```python
from build123d import *

# Parameters (mm, degrees)
SKETCH2_W           = 38.1
SKETCH2_H           = 38.1
SKETCH3_R           = 10
BOSS_EXTRUDE1_DEPTH = 38.1
FILLET1_R           = 40
SKETCH4_W           = 7.62
SKETCH4_H           = 59.936155674
SKETCH4_H_2         = 35.777885711
CUT_EXTRUDE1_DEPTH  = 60


with BuildPart() as part:
    # Sweep1: sweep along a path in Sketch1
    with BuildLine(Plane(origin=(0, 0, 0), x_dir=(0, 0, -1), z_dir=(1, 0, 0))) as sweep1_path:
        ThreePointArc((0, 0), (13.120743049, 34.179685259), (45.742360428, 50.8))
        Line((45.742360428, 50.8), (287.5, 76.2))
        Line((287.5, 76.2), (529.257639572, 50.8))
        ThreePointArc((529.257639572, 50.8), (561.879256951, 34.179685259), (575, 0))
    # Sketch2 → Sweep1 (sweep)
    with BuildSketch(Plane(origin=(0, 0, 0), x_dir=(1, 0, 0), z_dir=(0, 1, 0))):
        Rectangle(SKETCH2_W, SKETCH2_H)
    sweep(path=sweep1_path.line, transition=Transition.RIGHT)

    # Sketch3 → Boss-Extrude1 (add)
    with BuildSketch(Plane(origin=(19.05, 0, 0), x_dir=(0, 0, -1), z_dir=(1, 0, 0))):
        with BuildLine():
            ThreePointArc((317.5, 125), (267.165990691, 147.057381201), (285.064795638, 95.099000356))
            Line((285.064795638, 95.099000356), (287.5, 95.354852419))
            Line((287.5, 95.354852419), (289.935204362, 95.099000356))
            ThreePointArc((289.935204362, 95.099000356), (309.557381201, 104.665990691), (317.5, 125))
        make_face()
        with Locations((287.5, 125)):
            Circle(SKETCH3_R, mode=Mode.SUBTRACT)
    extrude(amount=-BOSS_EXTRUDE1_DEPTH)

    # Fillet1
    fillet1_edges = [part.edges().sort_by_distance(p)[0] for p in [
        (0, 95.099000356, -289.935204362),
        (0, 95.099000356, -285.064795638),
    ]]
    fillet(fillet1_edges, radius=FILLET1_R)

    # Sketch4 → Cut-Extrude1 (cut)
    with BuildSketch(Plane(origin=(0, 155, 0), x_dir=(1, 0, 0), z_dir=(0, 1, 0))):
        with Locations((-7.62, 287.5)):
            Rectangle(SKETCH4_W, SKETCH4_H)
        with Locations((-7.62, 335.357020692)):
            Rectangle(SKETCH4_W, SKETCH4_H_2)
        with Locations((7.62, 335.357020692)):
            Rectangle(SKETCH4_W, SKETCH4_H_2)
        with Locations((7.62, 287.5)):
            Rectangle(SKETCH4_W, SKETCH4_H)
        with Locations((7.62, 239.642979308)):
            Rectangle(SKETCH4_W, SKETCH4_H_2)
        with Locations((-7.62, 239.642979308)):
            Rectangle(SKETCH4_W, SKETCH4_H_2)
    extrude(amount=-CUT_EXTRUDE1_DEPTH, mode=Mode.SUBTRACT)


solid = part.part
```
Here's how the part is built. I have some questions about the finished solid (model axes, mm). A direction names the side the tool comes from. Round coordinates to 2 decimals unless told otherwise and drop trailing zeros. Order: outer loops, then holes, each group sorted by start corner. A loop starts at its lowest first (then second) coordinate and runs counter-clockwise, first axis right, second up. Notation, with made-up numbers: M 77.25,50 L 109.25,50 A30 ccw 109.25,80 Z; hole C -29.5,-19 d7. An arc over 180 degrees is marked long. Answer in a Markdown table with one row per item.
Item 1: Imagine slicing it at B-B, the plane z = -73.5. Write out the boundary of the cut face in (x, y).
A:
| item | result |
|---|---|
| outline | M -19.05,34.56 L 19.05,34.56 L 19.05,72.87 L -19.05,72.87 Z |
Item 2: Imagine slicing it at A-A, the plane y = 39. Write out the boundary of the cut face in (x, z), and give its area (3 significant figures).
A:
| item | result |
|---|---|
| outline | M -19.05,-582.21 L 19.05,-582.21 L 19.05,-459.25 L -19.05,-459.25 Z; M -19.05,-115.75 L 19.05,-115.75 L 19.05,7.21 L -19.05,7.21 Z |
| area | 9,370 mm2 |
Item 3: I'm going to push flat-ended pins straight in: pin 1 (6 mm diameter, centred on x = -4.5, y = 28, fed in from -Z); pin 2 (3 mm diameter, centred on x = 5.5, z = -74.5, fed in from +Y); pin 3 (12 mm diameter, centred on x = -11.5, z = -428.5, fed in from +Y). Where does each tip first touch, or does it pass through?
A:
| item | result |
|---|---|
| pin 1 | stops at z = -589.44 |
| pin 2 | stops at y = 73.13 |
| pin 3 | stops at y = 81.17 |
Item 4: Imagine slicing it at C-C, the plane y = 81.5. Write out the boundary of the cut face in (x, z).
A:
| item | result |
|---|---|
| outline | M -19.05,-419.37 L 19.05,-419.37 L 19.05,-155.63 L -19.05,-155.63 Z |
Item 5: Thinking about a two-plate mould opening in Y: for faces 1 (the face through (15.29, 131.76, -280.13)), 2 (the face through (0.05, 131.76, -280.13)), 3 (the face through (-0.27, 21.68, -547.5)), 4 (the face through (0.053, 154.993, -288.14)), which applies, +Y half, -Y half, draft (parallel to the pull), parting line (faces both ways), or undercut?
A:
| item | result |
|---|---|
| face 1 | undercut |
| face 2 | undercut |
| face 3 | -Y half |
| face 4 | +Y half |
Item 6: If I drill on L1, parallel to Y at x = -14, z = -287; L2, parallel to Z at x = 15.5, y = 9.5; L3, parallel to Y at x = -2, z = -493.5, over which ranges is the centre line in solid material (lowest first)? Write a range as from..to.
A:
| item | result |
|---|---|
| L1 | y = 56.99..115.01, 134.99..155 |
| L2 | z = -593.4..-554.51, -20.49..18.4 |
| L3 | y = 35.4..73.71 |
Item 7: For faces 5 (the face through (0, 0, 0)), 6 (the face through (11.43, 112, -287)), 7 (the face through (0.267, 44.626, -169.295)), which set-ups out of +Z, -Z, +X, -X, +Y, -Y let a thin tool reach every point of the face, with its end or its side?
A:
| item | result |
|---|---|
| face 5 | +Z, -Z, +X, -X, -Y |
| face 6 | +Z, -Z, +Y |
| face 7 | +X, -X, -Y |
